Could you check a few things on this model? Use its own coordinates, in mm. A direction names the side the tool comes from. Give positions to 0.01 mm unless a question says otherwise; leave off trailing zeros. Loops run counter-clockwise (first coordinate to the right, second up) from the corner with the lowest first, then second, coordinate; pieces in that order, holes last. Notation, with made-up numbers: (7.5, -4) - (32.5, -4) arc R14 ccw to (32.5, 15) - close; hole circle Ø5 at (0, -10). An arc over 180 degrees is marked (long way). Write each question's results on one line, items separated by ' | '. Start each with the question number.
1) If I drill on probe 1 along X at (y, z) = (1.5, 3.5); probe 2 along Z at (x, y) = (28, 0) (3 decimals); probe 3 along Z at (x, y) = (82, 1), over which ranges is the centre line in solid material (lowest first)? Write a range as [from, to].
2) If we mould it in two halves opening along Z, with no side actions, what happens to faces 4 (the face through (-4.742, -1.177, 2.077)), 5 (the face through (56.1, -1.5, 2.8)), 6 (the face through (114.3, 0, 0))? For each: +Z half, -Z half, draft (parallel to the pull), parting line (faces both ways), or undercut.
3) I want a section at A-A, the plane x = 29. Write out the boundary of the cut face in (y, z) (3 decimals).
4) On a 3-axis mill with a long thin cutter (end or side, diameter ignored), from which of +Z, -Z, +X, -X, +Y, -Y can I reach the whole of each face in a straight line? I mean faces 1 (the face through (-6.35, -2, 2)), 2 (the face through (-4.74, -1.21, -2.06)), 3 (the face through (0, 2, 3)). Say none if no direction works.
5) I'm going to push flat-ended pins straight in: pin 1 (5 mm diameter, centred on x = 66, z = 1.5, fed in from +Y) (3 decimals); pin 2 (1 mm diameter, centred on x = 16, z = 2.5, fed in from -Y); pin 3 (3 mm diameter, centred on x = 101, z = 1, fed in from -Y) (3 decimals). Where does each tip first touch, or does it pass through?
from build123d import *

# Parameters (mm, degrees)
SLOT_REACH    = 122.838
THREAD_R      = 0.635
CHAMFER1_SIZE = 0.75565
FILLET2_R     = 0.1778


with BuildPart() as part:
    # Sketch1 → Body (revolve)
    with BuildSketch(Plane.XY, mode=Mode.PRIVATE) as body_sk:
        Polygon((-1.710266667, 0), (114.3, 0), (114.3, 3.175), (88.9, 3.175), (85.7249, 3.175), (0, 3.175), (0, 4.7625), (-6.35, 4.7625), (-6.35, 2.756963005), (-3.302, 2.756963005), align=None)
    revolve(body_sk.sketch.rotate(Axis((-1.710266667, 0, 0), (1, 0, 0)), 180), axis=Axis((-1.710266667, 0, 0), (1, 0, 0)))

    # Slot: up to this cone (the profile starts inside it)
    slot_end = Plane(origin=(-6.35, 0, 0), z_dir=(-1, 0, 0)).offset(-4.639732333) * Cone(1.732e-06, 235.583136371, 136.0139862, align=(Align.CENTER, Align.CENTER, Align.MIN), mode=Mode.PRIVATE)
    # Sketch2 → Slot (add, up to the surface)
    with BuildSketch(Plane.ZY.offset(6.35), mode=Mode.PRIVATE) as slot_sk1:
        with BuildLine():
            ThreePointArc((1.378481503, -2.3876), (2.3876, -1.378481503), (2.756963005, 0))
            Line((2.756963005, 0), (1.378481503, -2.3876))
        make_face()
    slot_tool1 = extrude(slot_sk1.sketch, amount=-SLOT_REACH, mode=Mode.PRIVATE) & slot_end
    add(slot_tool1.solids().sort_by_distance((-6.35, -1.268114, 2.196438))[0])
    # Sketch2 → Slot (add, up to the surface)
    with BuildSketch(Plane.ZY.offset(6.35), mode=Mode.PRIVATE) as slot_sk2:
        with BuildLine():
            ThreePointArc((-1.378481503, -2.3876), (0, -2.756963005), (1.378481503, -2.3876))
            Line((1.378481503, -2.3876), (-1.378481503, -2.3876))
        make_face()
    slot_tool2 = extrude(slot_sk2.sketch, amount=-SLOT_REACH, mode=Mode.PRIVATE) & slot_end
    add(slot_tool2.solids().sort_by_distance((-6.35, -2.536228, 0))[0])
    # Sketch2 → Slot (add, up to the surface)
    with BuildSketch(Plane.ZY.offset(6.35), mode=Mode.PRIVATE) as slot_sk3:
        with BuildLine():
            ThreePointArc((-2.756963005, 0), (-2.3876, -1.378481503), (-1.378481503, -2.3876))
            Line((-1.378481503, -2.3876), (-2.756963005, 0))
        make_face()
    slot_tool3 = extrude(slot_sk3.sketch, amount=-SLOT_REACH, mode=Mode.PRIVATE) & slot_end
    add(slot_tool3.solids().sort_by_distance((-6.35, -1.268114, -2.196438))[0])
    # Sketch2 → Slot (add, up to the surface)
    with BuildSketch(Plane.ZY.offset(6.35), mode=Mode.PRIVATE) as slot_sk4:
        with BuildLine():
            Line((-2.756963005, 0), (-1.378481503, 2.3876))
            ThreePointArc((-1.378481503, 2.3876), (-2.3876, 1.378481503), (-2.756963005, 0))
        make_face()
    slot_tool4 = extrude(slot_sk4.sketch, amount=-SLOT_REACH, mode=Mode.PRIVATE) & slot_end
    add(slot_tool4.solids().sort_by_distance((-6.35, 1.268114, -2.196438))[0])
    # Sketch2 → Slot (add, up to the surface)
    with BuildSketch(Plane.ZY.offset(6.35), mode=Mode.PRIVATE) as slot_sk5:
        with BuildLine():
            Line((-1.378481503, 2.3876), (1.378481503, 2.3876))
            ThreePointArc((1.378481503, 2.3876), (0, 2.756963005), (-1.378481503, 2.3876))
        make_face()
    slot_tool5 = extrude(slot_sk5.sketch, amount=-SLOT_REACH, mode=Mode.PRIVATE) & slot_end
    add(slot_tool5.solids().sort_by_distance((-6.35, 2.536228, 0))[0])
    # Sketch2 → Slot (add, up to the surface)
    with BuildSketch(Plane.ZY.offset(6.35), mode=Mode.PRIVATE) as slot_sk6:
        with BuildLine():
            Line((1.378481503, 2.3876), (2.756963005, 0))
            ThreePointArc((2.756963005, 0), (2.3876, 1.378481503), (1.378481503, 2.3876))
        make_face()
    slot_tool6 = extrude(slot_sk6.sketch, amount=-SLOT_REACH, mode=Mode.PRIVATE) & slot_end
    add(slot_tool6.solids().sort_by_distance((-6.35, 1.268114, 2.196438))[0])

    # Thread
    thread_edges = [part.edges().sort_by_distance(p)[0] for p in [
        (-6.35, 4.7625, 0),
    ]]
    fillet(thread_edges, radius=THREAD_R)

    # Chamfer1
    chamfer1_edges = [part.edges().sort_by_distance(p)[0] for p in [
        (114.3, 3.175, 0),
    ]]
    chamfer(chamfer1_edges, length=CHAMFER1_SIZE)

    # Fillet2
    fillet2_edges = [part.edges().sort_by_distance(p)[0] for p in [
        (0, 3.175, 0),
    ]]
    fillet(fillet2_edges, radius=FILLET2_R)


solid = part.part
Answers:
1) probe 1: x = [-6.35, 0] | probe 2: z = [-3.175, 3.175] | probe 3: z = [-3.01, 3.01]
2) face 4: undercut | face 5: parting line | face 6: draft
3) outline: circle Ø6.35 at (0, 0)
4) face 1: +Z, -Z, -X, +Y, -Y | face 2: -X | face 3: +X
5) pin 1: stops at y = 3.175 | pin 2: stops at y = -2.47 | pin 3: stops at y = -3.175
